Model file for the job. Use its own axes, mm. A direction names the side the tool comes from. Give positions to 0.01 mm unless a question says otherwise; leave off trailing zeros. Write each loop counter-clockwise with the first axis right and the second up, starting at its lowest first coordinate (ties: lowest second). Pieces come first, ordered by that corner, then holes. Notation, with made-up numbers: (8.5, -26.5) - (52.5, -26.5) arc R16 ccw to (52.5, 4.5) - close; hole circle Ø4 at (41, -21). An arc over 180 degrees is marked (long way). One line per item, written item: value. Start each with the question number.
(1) Cut at D-D, the plane y = 3.75. List the corners of the cut face in (x, z), and give its area (3 significant figures).
(2) Cut at B-B, the plane z = 0. List the corners of the cut face in (x, y), and give its area (3 significant figures).
(3) Cut at C-C, the plane y = 5.75. List the corners of the cut face in (x, z).
(4) Probe L1, parallel to Z at x = 0, y = 3.25; L2, parallel to Y at x = 3.5, z = 0.25; L3, parallel to Y at x = -1.75, z = 0.5. List the from-to ranges inside material, lowest first.
(5) Cut at A-A, the plane x = 0. List the corners of the cut face in (y, z), and give its area (3 significant figures).
(6) 3-axis set-ups, long thin cutter, end or side, ignore diameter. For faces 4 (the face through (-5, 6.5, 0)), 5 (the face through (-5.3, 5.5, 0.6)): which of +Z, -Z, +X, -X, +Y, -Y reach the whole face in a straight line?
(7) Mould opens along X. For faces 1 (the face through (0, 1.5, 0)), 2 (the face through (-1.409, 2.725, 6.345)), 3 (the face through (4, 6.5, 0)) say: pulls with the +X half, pulls with the -X half, needs draft (parallel to the pull), parting line crosses it, or undercut.
(8) Drop flat-ended pins along their axis: P1, Ø4.5, axis at x = 0, z = -0.5, coming from the +Y side; P2, Ø1.5, axis at y = 3.5, z = -2.5, coming from the +X side; P3, Ø2, axis at y = 1.5, z = -4, coming from the +X side. Give the stop position or say it passes through.
from build123d import *

# Parameters (mm, degrees)
F0_R     = 6.5
F1_DEPTH = 4.5
F2_R     = 2
F3_DEPTH = 3
F4_R     = 1
F5_DEPTH = 2
F6_R     = 1
F8_ANGLE = -90


with BuildPart() as f1:
    # F0 (on Top) → F1 (new body)
    with BuildSketch(Plane.XY):
        Circle(F0_R)
    extrude(amount=F1_DEPTH)

    # F2 (on face) → F3 (cut)
    with BuildSketch(Plane.XY.offset(4.5)):
        Circle(F2_R)
    extrude(amount=-F3_DEPTH, mode=Mode.SUBTRACT)

    # F4 (on face) → F5 (join)
    with BuildSketch(Plane.XY.offset(4.5)):
        with Locations((-4.5, 0)):
            Circle(F4_R)
        with Locations((4.5, 0)):
            Circle(F4_R)
    extrude(amount=F5_DEPTH)

    # F6
    f6_edges = [f1.edges().sort_by_distance(p)[0] for p in [
        (-6.5, 0, 0),
    ]]
    fillet(f6_edges, radius=F6_R)


with BuildPart() as f1_1:
    # F8: moved
    add(f1.part.rotate(Axis((4.46189, 0, 0), (1, 0, 0)), F8_ANGLE))


solid = f1_1.part
Answers follow:
1. outline: circle Ø13 at (0, 0); hole circle Ø4 at (0, 0)
1. area: 120 mm²
2. outline: (-6.5, 1) arc R1 ccw to (-5.5, 0) - (5.5, 0) arc R1 ccw to (6.5, 1) - (6.5, 4.5) - (5.5, 4.5) - (5.5, 6.5) - (3.5, 6.5) - (3.5, 4.5) - (2, 4.5) - (2, 1.5) - (-2, 1.5) - (-2, 4.5) - (-3.5, 4.5) - (-3.5, 6.5) - (-5.5, 6.5) - (-5.5, 4.5) - (-6.5, 4.5) - close
2. area: 54.1 mm²
3. outline: circle Ø2 at (-4.5, 0); circle Ø2 at (4.5, 0)
4. L1: z = -6.5 to -2, 2 to 6.5
4. L2: y = 0 to 4.5
4. L3: y = 0 to 1.5
5. outline: (0, -5.5) arc R1 ccw to (1, -6.5) - (4.5, -6.5) - (4.5, -2) - (1.5, -2) - (1.5, 2) - (4.5, 2) - (4.5, 6.5) - (1, 6.5) arc R1 ccw to (0, 5.5) - close
5. area: 46.1 mm²
6. face 4: +Z, -Z, +X, -X, +Y
6. face 5: +Y
7. face 1: undercut
7. face 2: parting line crosses it
7. face 3: needs draft
8. P1: stops at y = 4.5
8. P2: stops at x = 6.26
8. P3: stops at x = 5.77
